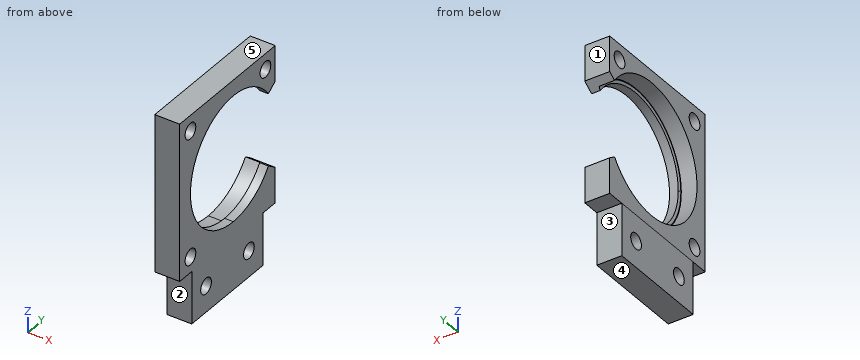
Autodesk Inventor part; units mm, degrees
ref_plane "Work Plane1" through (0, 0, 0) normal (-1, 0, 0) x (0, 0, 1)
ref_plane "YZ Plane" through (0, 0, 0) normal (1, 0, 0) x (0, 1, 0)
ref_plane "XZ Plane" through (0, 0, 0) normal (0, 1, 0) x (-1, 0, 0)
sketch "Sketch1" plane through (0, 0, 0) normal (1, 0, 0) x (0, 1, 0)
  line L0 (-15, 15) -> (15, 15)
  line L1 (15, 15) -> (15, -15)
  line L2 (15, -15) -> (-15, -15)
  line L3 (-15, -15) -> (-15, 15)
  line L4 (-15, 15) -> (15, -15) construction
  line L5 (15, 15) -> (-15, -15) construction
  point P0 (0, 0)
  dimension "d0" = 30
  dimension "d1" = 30
extrude "Extrusion1" add sketch "Sketch1" along normal blind 1.7695
sketch "Sketch2" plane through (1.7695, 0, 0) normal (1, 0, 0) x (0, 0, -1)
  circle A0 centre (0, 0) radius 12
  dimension "d4" = 24
extrude "Extrusion2" cut sketch "Sketch2" against normal up to next
sketch "Sketch3" plane through (0, 0, 0) normal (0, 0, 1) x (1, 0, 0)
  line L0 (1.7695, 15) -> (1.7695, -15)
  line L1 (1.7695, 0) -> (1.7695, -12.5584)
  line L2 (0.5, 0) -> (1.7695, 0)
  arc A0 (0.5, 0) -> (1.7695, -12.5584) centre (63.25, 0) ccw
  point P0 (0, 0)
  dimension "d7" = 12.5584
  dimension "d8" = 125.5
revolve "Revolution1" cut sketch "Sketch3" angle 360 about axis through (0.5, 0, 0) along (1, 0, 0)
sketch "Sketch4" plane through (1.7695, 0, 0) normal (1, 0, 0) x (0, 0, -1)
  circle A0 centre (0, 0) radius 12.7
  line L0 (-15, 15) -> (-15, -15)
  line L1 (-15, 15) -> (15, 15)
  line L2 (15, 15) -> (15, -15)
  line L3 (15, -15) -> (-15, -15)
  line L4 (-15, -15) -> (-15, 15)
  dimension "d10" = 25.4
extrude "Extrusion3" add sketch "Sketch4" along normal blind 3
ref_plane "Work Plane1" through (0, 0, 0) normal (-1, 0, 0) x (0, 0, 1)
mirror "Mirror1" about plane through (0, 0, 0) normal (-1, 0, 0) of "Extrusion1", "Extrusion2", "Revolution1", "Extrusion3"
sketch "Sketch8" plane through (4.7695, 0, 0) normal (1, 0, 0) x (0, 0, -1)
  circle A0 centre (12, -12) radius 1.5
  line L0 (-15, -15) -> (15, -15)
  line L1 (15, -15) -> (15, 15)
  circle A1 centre (-12, -12) radius 1.5
  circle A2 centre (-12, 9) radius 1.5
  line L2 (-15, 15) -> (-15, -15)
  line L3 (15, 15) -> (-15, 15)
  point P0 (0, 0)
  dimension "d30" = 3
  dimension "d31" = 3
  dimension "d32" = 3
  dimension "d33" = 3
  dimension "d34" = 3
  dimension "d35" = 3
  dimension "d36" = 6
extrude "Extrusion7" cut sketch "Sketch8" against normal up to surface (9.5391 mm away) contours A0 | A1 | A2
sketch "Sketch9" plane through (4.7695, 0, 0) normal (1, 0, 0) x (0, 0, -1)
  line L0 (0, 0) -> (-8.2274, 11.75)
  line L1 (-8.2274, 11.75) -> (-15, 11.75)
  line L2 (-15, 15) -> (-15, -15)
  line L3 (0, 0) -> (0, 15) construction
  line L4 (-15, 11.75) -> (-15, 15)
  line L5 (15, 15) -> (-15, 15)
  line L6 (0, 15) -> (-15, 15)
  line L7 (0, 0) -> (8.2274, 11.75)
  line L8 (8.2274, 11.75) -> (15, 11.75)
  line L9 (15, 15) -> (15, -15)
  line L10 (-15, 15) -> (15, 15)
  dimension "d39" = 35
  dimension "d42" = 3.25
extrude "Extrusion8" cut sketch "Sketch9" against normal up to surface (9.5391 mm away)
sketch "Sketch11" plane through (4.7695, -15, -15) normal (0, 0, -1) x (-1, 0, 0)
  line L0 (9.5391, 0) -> (9.5391, 26.75)
  line L1 (0, 0) -> (9.5391, 26.75) construction
  line L2 (0, 26.75) -> (9.5391, 26.75)
  line L3 (0, 26.75) -> (9.5391, 0) construction
  line L4 (0, 0) -> (0, 26.75)
  line L5 (9.5391, 3.375) -> (0, 3.375)
  line L6 (0, 3.375) -> (0, 23.375)
  line L7 (0, 23.375) -> (9.5391, 23.375)
  line L8 (9.5391, 23.375) -> (9.5391, 3.375)
  line L9 (9.5391, 3.375) -> (0, 23.375) construction
  line L10 (0, 3.375) -> (9.5391, 23.375) construction
  point P0 (4.7695, 15)
  point P1 (4.7695, 13.375)
  dimension "d46" = 20
extrude "Extrusion10" add sketch "Sketch11" along normal blind 10 contours L5 L4 L7 L0
sketch "Sketch12" plane through (-4.7695, -15, -15) normal (-1, 0, 0) x (0, 0, 1)
  circle A0 centre (-5, 19.375) radius 1.5
  circle A1 centre (-5, 7.375) radius 1.5
  line L0 (0, 3.375) -> (-10, 3.375)
  line L1 (0, 23.375) -> (-10, 23.375)
  point P0 (15, 15)
  dimension "d49" = 4
  dimension "d50" = 5
  dimension "d51" = 4
  dimension "d52" = 5
  dimension "d53" = 3
extrude "Extrusion11" cut sketch "Sketch12" against normal up to surface (9.5391 mm away)
sketch "Sketch13" plane through (4.7695, -15, -15) normal (0, -1, 0) x (1, 0, 0)
  line L0 (-9.5391, 30) -> (0, 30)
  line L1 (-4.7695, 30) -> (-4.7695, -10)
  line L2 (0, -10) -> (-9.5391, -10)
  point P0 (-4.7695, 15)
split body "Split2" sketch "Sketch13" result one side removed curves L1 removed pieces at (0.5, -13.971, -0.4809)
equation "\"d37\" = d32"
properties part number "LargeLensHolderP1S2" material "Acetal Resin, Black"
Build history of the part. All positions in model axes, mm. Face numbers are marked on the shaded views. A direction names the side the tool comes from. Round coordinates to 2 decimals unless told otherwise and drop trailing zeros. Write each loop counter-clockwise with the first axis right and the second up, starting at its lowest first coordinate (ties: lowest second). Pieces come first, ordered by that corner, then holes. Notation, with made-up numbers: M -37.75,77.25 L -11.75,77.25 A32 cw -11.75,105.25 Z; hole C -5,32 d3. An arc over 180 degrees is marked long. Answer as a JSON object with one key per item and string values. Group by question number.
(1) Cut at A-A (z = -20). Give the cut face in (x, y) (1 decimal), and give its area (3 significant figures).
(2) Flat gauge pins, fed straight in: pin 1 (1.4 mm diameter, centred on x = -2.5, z = -17.5, fed in from -Y) (3 decimals); pin 2 (2.5 mm diameter, centred on y = 4.375, z = -20, fed in from -X); pin 3 (1.7 mm diameter, centred on x = -2, y = -13, fed in from -Z). Where does each tip first touch, or does it go through?
(3) Cut at C-C (y = 9). Give the number of separate pieces and of enclosed holes in the cut face, and give its area (3 significant figures).
(4) Mould opens along Z. For the marked faces 3, 4 and 5 say: pulls with the +Z half, pulls with the -Z half, needs draft (parallel to the pull), parting line crosses it, or undercut.
(5) Drill centre lines: L1, parallel to Y at x = -2.1, z = -20.5 (3 decimals); L2, parallel to Z at x = -0.6, y = 0; L3, parallel to Z at x = -2.7, y = 8.5. Where is each one in solid material? Low to high.
(6) Which spindle directions (+Z, -Z, +X, -X, +Y, -Y) get a long thin tool onto all of the face, cutting with end or side? Do the marked faces 1 and 2. Say none if no direction does.
(7) Cut at B-B (x = -2.25). Give the cut face in (y, z) (3 decimals).
Responses:
{
 "1": {"outline": "M -4.8,-11.6 L 0,-11.6 L 0,-9.1 L -4.8,-9.1 Z; M -4.8,-6.1 L 0,-6.1 L 0,2.9 L -4.8,2.9 Z; M -4.8,5.9 L 0,5.9 L 0,8.4 L -4.8,8.4 Z", "area": "66.8 mm2"},
 "2": {"pin 1": "stops at y = -11.625", "pin 2": "passes through", "pin 3": "stops at z = -15"},
 "3": {"separate pieces": "3", "enclosed holes": "0", "area": "46.8 mm2"},
 "4": {"face 3": "needs draft", "face 4": "pulls with the -Z half", "face 5": "pulls with the +Z half"},
 "5": {"L1": "y = -11.625 to -9.039, -6.211 to 2.961, 5.789 to 8.375", "L2": "z = -25 to -12, 12 to 15", "L3": "z = -15 to -9.44, 9.44 to 10.59, 13.41 to 15"},
 "6": {"face 1": "+Z, -Z, +X, -X, +Y", "face 2": "-Z, +X, -X, -Y"},
 "7": {"outline": "M -15,-15 L -11.625,-15 L -11.625,-25 L 8.375,-25 L 8.375,-15 L 11.75,-15 L 11.75,-8.227 L 10.403,-7.284 A12.7 cw long 10.403,7.284 L 11.75,8.227 L 11.75,15 L -15,15 Z; hole C -12,-12 d3; hole C -12,12 d3; hole C -7.625,-20 d3; hole C 4.375,-20 d3; hole C 9,12 d3"}
}
